Part model, mm, in its own coordinate system. A direction names the side the tool comes from. Coordinates: 2 decimals unless noted, no trailing zeros. Loops run counter-clockwise (first coordinate to the right, second up) from the corner with the lowest first, then second, coordinate; pieces in that order, holes last. Notation, with made-up numbers: (37.25, 29) - (91.25, 29) arc R19 cw to (91.25, 40) - close; hole circle Ø8 at (69.25, 85). An arc over 180 degrees is marked (long way). Use a Markdown table: item, result. Add a question column.
1. Band-saw the part on B-B, the plane x = 0. Give the cut face in (y, z).
2. Band-saw the part on C-C, the plane z = 3. Give the cut face in (x, y).
3. Wall check: probe 1 along X at (y, z) = (4.1, 3); probe 2 along X at (y, z) = (-1.75, 3.5); probe 3 along X at (y, z) = (0, 1.9). Give the ranges that are in metal, low to high. Write a range as [from, to].
4. Band-saw the part on D-D, the plane z = 5. Give the cut face in (x, y), plus the area to 3 significant figures.
5. Drop flat-ended pins along their axis: pin 1 (1 mm diameter, centred on x = -10.5, z = 3, fed in from +Y); pin 2 (1.8 mm diameter, centred on x = -11, z = 4, fed in from -Y); pin 3 (3 mm diameter, centred on x = -10, z = 2, fed in from -Y). Give the stop position or say it passes through.
6. Band-saw the part on A-A, the plane y = -3. Give the cut face in (x, z), plus the area to 3 significant figures.
7. Pull direction X, two halves, no side cores. Call faces 1 (the cylindrical face through (-14.473, -3.965, 2.93)), 2 (the cylindrical face through (7.739, 7.817, 2.958)), 3 (the flat face through (-15, -6.5, 3)): pulls with the +X half, pulls with the -X half, needs draft (parallel to the pull), parting line crosses it, or undercut.
8. 3-axis set-ups, long thin cutter, end or side, ignore diameter. For faces 4 (the flat face through (-11, -6.5, 3)), 5 (the flat face through (-11, 6.5, 3)), 6 (the flat face through (-10, 1.5, 3)): which of +Z, -Z, +X, -X, +Y, -Y reach the whole face in a straight line?
Autodesk Inventor part; units mm, degrees
ref_plane "YZ Plane" through (0, 0, 0) normal (1, 0, 0) x (0, 1, 0)
ref_plane "XZ Plane" through (0, 0, 0) normal (0, 1, 0) x (-1, 0, 0)
ref_plane "XY Plane" through (0, 0, 0) normal (0, 0, 1) x (1, 0, 0)
sketch "スケッチ1" plane through (0, 0, 0) normal (0, 0, 1) x (1, 0, 0)
  circle A0 centre (3.5267, 4.8541) radius 1.25
  circle A1 centre (3.5267, -4.8541) radius 1.25
  line L0 (3.5267, 4.8541) -> (0, 0) construction
  line L1 (0, 0) -> (3.5267, -4.8541) construction
  line L2 (0, 0) -> (7.2054, 0) construction
  circle A2 centre (0, 0) radius 4.05
  arc A3 (-8.8741, 6.5) -> (-8.8741, -6.5) centre (0, 0) ccw construction
  line L3 (-8.8741, 6.5) -> (-12.3356, 6.5)
  line L4 (-16.8741, 6.5) -> (-16.8741, 1.5)
  line L5 (-16.8741, 1.5) -> (-3.762, 1.5)
  line L6 (-3.762, -1.5) -> (-16.8741, -1.5)
  line L7 (-16.8741, -1.5) -> (-16.8741, -6.5)
  line L8 (-16.8741, -6.5) -> (-13.4126, -6.5)
  line L9 (-4.5826, 10) -> (4.5826, 10)
  line L10 (-4.5826, -10) -> (4.5826, -10)
  line L11 (10, 4.5826) -> (10, -4.5826)
  circle A4 centre (0, 0) radius 10 construction
  arc A5 (-12.3356, 6.5) -> (-13.4126, 6.5) centre (-12.8741, 7.9) ccw construction
  arc A6 (-12.3356, -6.5) -> (-13.4126, -6.5) centre (-12.8741, -7.9) ccw
  arc A7 (-4.5826, 10) -> (-8.8741, 6.5) centre (0, 0) ccw
  arc A8 (4.5826, 10) -> (-4.5826, 10) centre (0, 0) ccw construction
  arc A9 (10, 4.5826) -> (4.5826, 10) centre (0, 0) ccw
  arc A10 (10, -4.5826) -> (10, 4.5826) centre (0, 0) ccw construction
  arc A11 (4.5826, -10) -> (10, -4.5826) centre (0, 0) ccw
  arc A12 (-4.5826, -10) -> (4.5826, -10) centre (0, 0) ccw construction
  arc A13 (-8.8741, -6.5) -> (-4.5826, -10) centre (0, 0) ccw
  arc A14 (-13.4126, 6.5) -> (-12.3356, 6.5) centre (-12.8741, 7.9) ccw
  line L12 (-13.4126, 6.5) -> (-16.8741, 6.5)
  line L13 (-12.3356, 6.5) -> (-13.4126, 6.5) construction
  arc A15 (-13.4126, -6.5) -> (-12.3356, -6.5) centre (-12.8741, -7.9) ccw construction
  line L14 (-13.4126, -6.5) -> (-12.3356, -6.5) construction
  line L15 (-12.3356, -6.5) -> (-8.8741, -6.5)
  dimension "d0" = 2.5
  dimension "d1" = 2.5
  dimension "d2" = 6
  dimension "d3" = 6
  dimension "d4" = 108
  dimension "d5" = 54
  dimension "d6" = 8.1
  dimension "d7" = 22
  dimension "d8" = 5
  dimension "d9" = 5
  dimension "d10" = 20
  dimension "d11" = 3
  dimension "d12" = 1.5
  dimension "d13" = 8
  dimension "d14" = 3
  dimension "d15" = 3
  dimension "d16" = 1.4
  dimension "d17" = 1.4
  dimension "d18" = 4
  dimension "d19" = 4
extrude "押し出し1" add sketch "スケッチ1" along normal blind 6 contours A2 L5 L4 L12 A14 L3 A7 L9 A9 L11 A11 L10 A13 L15 A6 L8 L7 L6
sketch "スケッチ2" plane through (-16.8741, 6.5, 0) normal (0, 1, 0) x (1, 0, 0)
  circle A0 centre (4, -3) radius 1.6
  line L0 (4.5385, 0) -> (3.4615, 0)
  point P0 (16.8741, 0)
  point P1 (4, 0)
  dimension "d22" = 3.2
  dimension "d23" = 3
extrude "押し出し2" cut sketch "スケッチ2" against normal through all
equation "\"d5\" = 0.5 * d4"
equation "\"d12\" = 0.5 * d11"
properties part number "ギア固定具1"
Geometry check:
| question | item | result |
|---|---|---|
| 1 | outline | (-10, 0) - (-4.05, 0) - (-4.05, 6) - (-10, 6) - close; (4.05, 0) - (10, 0) - (10, 6) - (4.05, 6) - close |
| 2 | outline | (-16.87, -6.5) - (-14.47, -6.5) - (-14.47, -1.5) - (-16.87, -1.5) - close; (-16.87, 1.5) - (-14.47, 1.5) - (-14.47, 6.5) - (-16.87, 6.5) - close; (-11.27, -6.5) - (-8.87, -6.5) arc R11 ccw to (-4.58, -10) - (4.58, -10) arc R11 ccw to (10, -4.58) - (10, 4.58) arc R11 ccw to (4.58, 10) - (-4.58, 10) arc R11 ccw to (-8.87, 6.5) - (-11.27, 6.5) - (-11.27, 1.5) - (-3.76, 1.5) arc R4.05 cw (long way) to (-3.76, -1.5) - (-11.27, -1.5) - close; hole circle Ø2.5 at (3.53, -4.85); hole circle Ø2.5 at (3.53, 4.85) |
| 3 | probe 1 | x = [-16.87, -14.47], [-11.27, 2.53], [4.52, 10] |
| 3 | probe 2 | x = [-16.87, -14.39], [-11.35, -3.65], [3.65, 10] |
| 3 | probe 3 | x = [4.05, 10] |
| 4 | outline | (-16.87, -6.5) - (-13.41, -6.5) arc R1.5 cw to (-12.34, -6.5) - (-8.87, -6.5) arc R11 ccw to (-4.58, -10) - (4.58, -10) arc R11 ccw to (10, -4.58) - (10, 4.58) arc R11 ccw to (4.58, 10) - (-4.58, 10) arc R11 ccw to (-8.87, 6.5) - (-12.34, 6.5) arc R1.5 cw to (-13.41, 6.5) - (-16.87, 6.5) - (-16.87, 1.5) - (-3.76, 1.5) arc R4.05 cw (long way) to (-3.76, -1.5) - (-16.87, -1.5) - close; hole circle Ø2.5 at (3.53, -4.85); hole circle Ø2.5 at (3.53, 4.85) |
| 4 | area | 347 mm^2 |
| 5 | pin 1 | stops at y = 6.5 |
| 5 | pin 2 | stops at y = -6.5 |
| 5 | pin 3 | stops at y = -6.98 |
| 6 | outline | (-16.87, 0) - (-2.72, 0) - (-2.72, 6) - (-16.87, 6) - close; (2.72, 0) - (10, 0) - (10, 6) - (2.72, 6) - close; hole circle Ø3.2 at (-12.87, 3) |
| 6 | area | 121 mm^2 |
| 7 | face 1 | undercut |
| 7 | face 2 | pulls with the +X half |
| 7 | face 3 | needs draft |
| 8 | face 4 | +Z, -Z, -X, -Y |
| 8 | face 5 | +Z, -Z, -X, +Y |
| 8 | face 6 | +Z, -Z, -X |
